Input: part model. Units: mm. Frame: model coordinates. Face numbers are marked on the shaded views. A direction names the side the tool comes from. Coordinates: 2 decimals unless noted, no trailing zeros. Loops run counter-clockwise (first coordinate to the right, second up) from the corner with the lowest first, then second, coordinate; pieces in that order, holes last. Notation, with made-up numbers: (-3.5, 63.25) - (47.5, 63.25) arc R15 cw to (47.5, 91.25) - close; hole circle Ø9 at (-10, 57.5). An arc over 180 degrees is marked (long way). Use a Markdown table: item, result. Add a question column.
1. Contact query for flat-ended pins moving along their axis: P1, Ø14, axis at x = -18, y = 14, coming from the +Z side; P2, Ø6.5, axis at x = 0, y = 35, coming from the -Z side; P3, Ø5, axis at x = 22, z = 7, coming from the -Y side. Output: stop coordinate, or through.
2. Ray query, L1, parallel to Y at x = 0, z = 3; L2, parallel to X at y = 15, z = 1; L3, parallel to Y at x = -1, z = 10. Return the intervals inside material, ascending. Write a range as [from, to].
3. Section query B-B on z = -5. Return the cut outline in (x, y), then the cut area to 3 significant figures.
4. Access query for the marked faces 5 and 6. Directions: +Z, -Z, +X, -X, +Y, -Y. A direction counts if a zero-diameter tool reaches every point of the face in a straight line with its end or side. Return the directions, or none.
5. Section query D-D on y = 13. Return the cut outline in (x, z).
6. Section query A-A on y = 25.5. Return the cut outline in (x, z).
7. Draft query along Y for the marked faces 1, 2, 3 and 4. Return one class per face: released by +Y, released by -Y, zero draft, split by the parting line, or undercut.
8. Section query C-C on x = 17.5. Return the cut outline in (y, z).
```python
from build123d import *

# Parameters (mm, degrees)
F1_DEPTH = 16
F2_R     = 2.0625
F3_DEPTH = 8
F5_DEPTH = 8


with BuildPart() as f1:
    # F0 (on Top) → F1 (new body, symmetric)
    with BuildSketch(Plane.XY):
        with BuildLine():
            Line((-45, 3.500000108), (-45, 0))
            Line((-45, 0), (19.080892972, 0))
            ThreePointArc((19.080892972, 0), (29.3414972718, 1.8092213764), (38.3645212626, 7.0186667064))
            Line((38.3645212626, 7.0186667064), (47.8763038889, 15))
            Line((47.8763038889, 15), (45.6265471856, 17.6811556337))
            Line((45.6265471856, 17.6811556337), (36.1147645593, 9.6998223401))
            ThreePointArc((36.1147645593, 9.6998223401), (28.1444267332, 5.0981456507), (19.080892972, 3.500000108))
            Line((19.080892972, 3.500000108), (-45, 3.500000108))
        make_face()
    extrude(amount=F1_DEPTH, both=True)

    # F2 (on Top) → F3 (join)
    with BuildSketch(Plane.XY):
        with BuildLine():
            Line((-7.6244007781, 38.7574609479), (-25, 3.500000108))
            Line((-25, 3.500000108), (-20.5406331606, 3.500000108))
            Line((-20.5406331606, 3.500000108), (-7.2241458503, 30.5209692194))
            ThreePointArc((-7.2241458503, 30.5209692194), (-8.4899813452, 34.5874266639), (-7.6244007781, 38.7574609479))
        make_face()
        with BuildLine():
            ThreePointArc((6.1274973095, 40.8909911493), (-1.3031376668, 43.3995138086), (-7.6244007781, 38.7574609479))
            ThreePointArc((-7.6244007781, 38.7574609479), (-8.4899813452, 34.5874266639), (-7.2241458503, 30.5209692194))
            ThreePointArc((-7.2241458503, 30.5209692194), (1.3031376668, 26.6004861914), (8.2416799056, 32.9204057285))
            ThreePointArc((8.2416799056, 32.9204057285), (8.4351727664, 33.952211662), (8.5, 35))
            ThreePointArc((8.5, 35), (7.8845966013, 38.1753954769), (6.1274973095, 40.8909911493))
        make_face()
        with Locations((0, 35)):
            Circle(F2_R, mode=Mode.SUBTRACT)
        with BuildLine():
            Line((36.1147645593, 9.6998223401), (6.1274973095, 40.8909911493))
            ThreePointArc((6.1274973095, 40.8909911493), (7.8845966013, 38.1753954769), (8.5, 35))
            ThreePointArc((8.5, 35), (8.4351727664, 33.952211662), (8.2416799056, 32.9204057285))
            Line((8.2416799056, 32.9204057285), (32.8294657363, 7.3454918124))
            ThreePointArc((32.8294657363, 7.3454918124), (34.517066012, 8.45993138), (36.1147645593, 9.6998223401))
        make_face()
    extrude(amount=F3_DEPTH)

    # F4 (on face) → F5 (join)
    with BuildSketch(Plane.XY.offset(8)):
        with BuildLine():
            ThreePointArc((8.2416799056, 32.9204057285), (8.4351727664, 33.952211662), (8.5, 35))
            ThreePointArc((8.5, 35), (7.8845966013, 38.1753954769), (6.1274973095, 40.8909911493))
            ThreePointArc((6.1274973095, 40.8909911493), (-1.3031376668, 43.3995138086), (-7.6244007781, 38.7574609479))
            ThreePointArc((-7.6244007781, 38.7574609479), (-8.4899813452, 34.5874266639), (-7.2241458503, 30.5209692194))
            ThreePointArc((-7.2241458503, 30.5209692194), (1.3031376668, 26.6004861914), (8.2416799056, 32.9204057285))
        make_face()
        Polygon((-6.9859382572, 35), (-3.4929691286, 41.05), (3.4929691286, 41.05), (6.9859382572, 35), (3.4929691286, 28.95), (-3.4929691286, 28.95), align=None, mode=Mode.SUBTRACT)
    extrude(amount=F5_DEPTH)


solid = f1.part
```
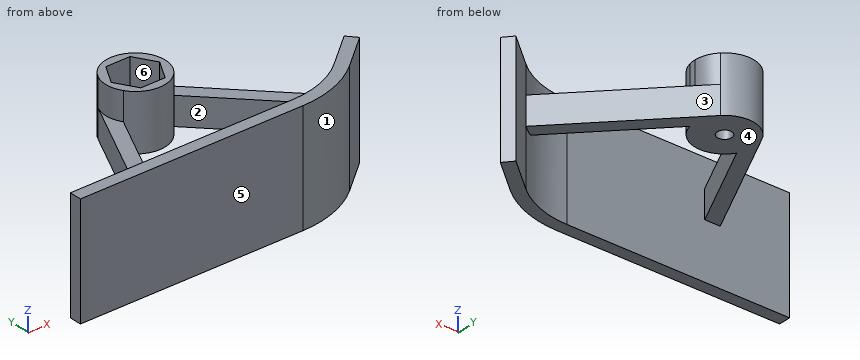
Resolved:
| question | item | result |
|---|---|---|
| 1 | P1 | z = 8 |
| 1 | P2 | z = 0 |
| 1 | P3 | y = 0 |
| 2 | L1 | [0, 3.5], [26.5, 32.94], [37.06, 43.5] |
| 2 | L2 | [-19.33, -14.87], [25.47, 31.02], [42.43, 47.88] |
| 2 | L3 | [0, 3.5], [26.56, 28.95], [41.05, 43.44] |
| 3 | outline | (-45, 0) - (19.08, 0) arc R30 ccw to (38.36, 7.02) - (47.88, 15) - (45.63, 17.68) - (36.11, 9.7) arc R26.5 cw to (19.08, 3.5) - (-45, 3.5) - close |
| 3 | area | 337 mm² |
| 4 | face 5 | +Z, -Z, +X, -X, -Y |
| 4 | face 6 | +Z |
| 5 | outline | (-20.32, 0) - (-15.86, 0) - (-15.86, 8) - (-20.32, 8) - close; (27.39, 0) - (32.94, 0) - (32.94, 8) - (27.39, 8) - close; (40.05, -16) - (45.49, -16) - (45.49, 16) - (40.05, 16) - close |
| 6 | outline | (-14.16, 0) - (-9.7, 0) - (-9.7, 8) - (-14.16, 8) - close; (15.38, 0) - (20.92, 0) - (20.92, 8) - (15.38, 8) - close |
| 7 | face 1 | released by -Y |
| 7 | face 2 | undercut |
| 7 | face 3 | released by +Y |
| 7 | face 4 | zero draft |
| 8 | outline | (0, -16) - (3.5, -16) - (3.5, 16) - (0, 16) - close; (23.29, 0) - (29.06, 0) - (29.06, 8) - (23.29, 8) - close |
